```python
from build123d import *
from OCP.BRepFilletAPI import BRepFilletAPI_MakeChamfer

# Parameters (mm, degrees)
SKETCH1_R           = 1.5
BOSS_EXTRUDE1_DEPTH = 50
SKETCH2_W           = 6
SKETCH2_H           = 50
BOSS_EXTRUDE2_DEPTH = 50
CHAMFER1_SIZE       = 50
CHAMFER1_SIZE2      = 20
SKETCH4_W           = 6
SKETCH4_H           = 3
BOSS_EXTRUDE3_DEPTH = 6
SKETCH5_R           = 1.5
CUT_EXTRUDE1_DEPTH  = 65.747586828
CHAMFER2_SIZE       = 1
CHAMFER2_SIZE2      = 1.795054936
FILLET1_R           = 2
CUT_EXTRUDE2_DEPTH  = 6
CUT_EXTRUDE3_DEPTH  = 78.569323834
BOSS_EXTRUDE5_DEPTH = 6
CUT_EXTRUDE4_DEPTH  = 78.569323834
FILLET2_R           = 10


with BuildPart() as part:
    # Sketch1 → Boss-Extrude1 (new body)
    with BuildSketch(Plane(origin=(0, 0, 0), x_dir=(1, 0, 0), z_dir=(0, 1, 0))):
        with BuildLine():
            Line((0, 3), (-3, 3))
            Line((-3, 3), (-3, -3))
            Line((-3, -3), (0, -3))
            ThreePointArc((0, -3), (3, 0), (0, 3))
        make_face()
        with Locations(Location((0, 0, 0), (0, 0, 270))):
            Circle(SKETCH1_R, mode=Mode.SUBTRACT)
    extrude(amount=BOSS_EXTRUDE1_DEPTH)

    # Sketch2 → Boss-Extrude2 (add)
    with BuildSketch(Plane.ZY.offset(3)):
        with Locations((0, 25)):
            Rectangle(SKETCH2_W, SKETCH2_H)
    extrude(amount=BOSS_EXTRUDE2_DEPTH)

    # Chamfer1: one chamfer whose edges measure the first distance from different faces: ONE call of the kernel's chamfer builder (chamfer() names one face for all edges)
    chamfer1_edges_1 = [part.edges().sort_by_distance(p)[0] for p in [
        (-53, 50, 0),
    ]]
    chamfer1_side_1 = [part.faces().sort_by_distance(p)[0] for p in [
        (-25.86838725, 50, 0),
    ]]
    chamfer1_edges_2 = [part.edges().sort_by_distance(p)[0] for p in [
        (-53, 0, 0),
    ]]
    chamfer1_side_2 = [part.faces().sort_by_distance(p)[0] for p in [
        (-25.86838725, 0, 0),
    ]]
    chamfer1 = BRepFilletAPI_MakeChamfer(part.part.solid().wrapped)
    for e in chamfer1_edges_1:
        chamfer1.Add(CHAMFER1_SIZE, CHAMFER1_SIZE2, e.wrapped, chamfer1_side_1[0].wrapped)  # the first distance lies on this face
    for e in chamfer1_edges_2:
        chamfer1.Add(CHAMFER1_SIZE, CHAMFER1_SIZE2, e.wrapped, chamfer1_side_2[0].wrapped)  # the first distance lies on this face
    add(Compound.cast(chamfer1.Shape()), mode=Mode.REPLACE)

    # Sketch4 → Boss-Extrude3 (add)
    with BuildSketch(Plane.ZY.offset(53)):
        with Locations((0, 25)):
            Rectangle(SKETCH4_W, SKETCH4_H)
    extrude(amount=BOSS_EXTRUDE3_DEPTH)

    # Sketch5 → Cut-Extrude1 (cut, through all)
    with BuildSketch(Plane.XZ.offset(-23.5)):
        with Locations(Location((-56, 0, 0), (0, 0, 270))):
            Circle(SKETCH5_R)
    extrude(amount=-CUT_EXTRUDE1_DEPTH, mode=Mode.SUBTRACT)

    # Chamfer2: one chamfer whose edges measure the first distance from different faces: ONE call of the kernel's chamfer builder (chamfer() names one face for all edges)
    chamfer2_edges_1 = [part.edges().sort_by_distance(p)[0] for p in [
        (-53, 30, 0),
    ]]
    chamfer2_side_1 = [part.faces().sort_by_distance(p)[0] for p in [
        (-28, 40, 0),
    ]]
    chamfer2_edges_2 = [part.edges().sort_by_distance(p)[0] for p in [
        (-53, 20, 0),
    ]]
    chamfer2_side_2 = [part.faces().sort_by_distance(p)[0] for p in [
        (-28, 10, 0),
    ]]
    chamfer2 = BRepFilletAPI_MakeChamfer(part.part.solid().wrapped)
    for e in chamfer2_edges_1:
        chamfer2.Add(CHAMFER2_SIZE, CHAMFER2_SIZE2, e.wrapped, chamfer2_side_1[0].wrapped)  # the first distance lies on this face
    for e in chamfer2_edges_2:
        chamfer2.Add(CHAMFER2_SIZE, CHAMFER2_SIZE2, e.wrapped, chamfer2_side_2[0].wrapped)  # the first distance lies on this face
    add(Compound.cast(chamfer2.Shape()), mode=Mode.REPLACE)

    # Fillet1
    fillet1_edges = [part.edges().sort_by_distance(p)[0] for p in [
        (-59, 25, 3),
        (-59, 25, -3),
    ]]
    fillet(fillet1_edges, radius=FILLET1_R)

    # Sketch6 → Cut-Extrude2 (cut)
    with BuildSketch(Plane.XY.offset(3)):
        Polygon((-7.907152331, 5), (-5.507152331, 5), (-5.507152331, 45), (-7.907152331, 45), (-47.164370978, 29.297112541), (-47.907152331, 27.563956051), (-47.907152331, 22.436043949), (-47.164370978, 20.702887459), align=None)
    extrude(amount=-CUT_EXTRUDE2_DEPTH, mode=Mode.SUBTRACT)

    # Sketch7 → Cut-Extrude3 (cut, through all)
    with BuildSketch(Plane.XY.offset(3)):
        Polygon((-53, 28.204945064), (-53, 26.5), (-47.907152331, 26.5), (-47.907152331, 27.563956051), (-47.164370978, 29.297112541), (-25.810496084, 37.838662499), (-14.112413915, 45.555034434), (-52.071523309, 30.371390676), align=None)
        Polygon((-47.907152331, 23.5), (-53, 23.5), (-53, 21.795054936), (-52.071523309, 19.628609324), (-14.112413915, 4.444965566), (-25.810496084, 12.161337501), (-47.164370978, 20.702887459), (-47.907152331, 22.436043949), align=None)
    extrude(amount=-CUT_EXTRUDE3_DEPTH, mode=Mode.SUBTRACT)


with BuildPart() as cut_extrude3_piece_1:
    # of the separate pieces the step leaves, piece 1, a body of its own (cut_extrude3_pieces)
    add(part.part.solids().sort_by_distance((-3, 50, -3))[0])



with BuildPart() as cut_extrude3_piece_2:
    # of the separate pieces the step leaves, piece 2, a body of its own (cut_extrude3_pieces)
    add(part.part.solids().sort_by_distance((-57, 26.5, -3))[0])


with BuildPart() as cut_extrude3_piece_1_1:
    add(cut_extrude3_piece_1.part)

    add(cut_extrude3_piece_2.part)  # Boss-Extrude5 merges Cut-Extrude3 piece 2
    # Sketch7<3> → Boss-Extrude5 (add)
    with BuildSketch(Plane.XY.offset(3)):
        Polygon((-43, 26.5), (-53, 26.5), (-53, 23.5), (-43, 23.5), (-14.112413915, 4.444965566), (-3, 0), (-3, 50), (-14.112413915, 45.555034434), align=None)
    extrude(amount=-BOSS_EXTRUDE5_DEPTH)

    # Sketch8 → Cut-Extrude4 (cut, through all)
    with BuildSketch(Plane.XY.offset(3)):
        Polygon((-35.341555741, 26.05), (-15.120245482, 39.388524104), (-7.341555741, 42.5), (-5.241555741, 42.5), (-5.241555741, 7.5), (-7.341555741, 7.5), (-15.120245482, 10.611475896), (-35.341555741, 23.95), align=None)
    extrude(amount=-CUT_EXTRUDE4_DEPTH, mode=Mode.SUBTRACT)

    # Fillet2
    fillet2_edges = [cut_extrude3_piece_1_1.edges().sort_by_distance(p)[0] for p in [
        (-43, 23.5, 0),
        (-43, 26.5, 0),
    ]]
    fillet(fillet2_edges, radius=FILLET2_R)


solid = cut_extrude3_piece_1_1.part
```
Design review of the part built by this model. Coordinates are the model's own, in mm. A direction names the side the tool comes from. Give positions to 0.01 mm unless a question says otherwise; leave off trailing zeros. Write each loop counter-clockwise with the first axis right and the second up, starting at its lowest first coordinate (ties: lowest second). Pieces come first, ordered by that corner, then holes. Notation, with made-up numbers: (39, -29.75) -> (60, -29.75) arc R23 ccw to (60, -11.75) -> close; hole circle Ø8 at (-24, -27.5). An arc over 180 degrees is marked (long way). Answer in a Markdown table with one row per item.
(1) Consider section D-D (y = 44.5). State the section outline as (x, z) points, then the cut area to 3 significant figures.
Results:
| item | result |
|---|---|
| outline | (-15.71, -3) -> (0, -3) arc R3 ccw to (0, 3) -> (-15.71, 3) -> close; hole circle Ø3 at (0, 0) |
| area | 101 mm2 |
(2) Mouldability with a two-part tool opening along Y and no side actions: class faces 5 (the flat face through (-25.372, 32.626, 0.042)), 6 (the flat face through (-8.63, 47.75, -0.04)), 7 (the flat face through (-59, 25, 0)) as +Y half, -Y half, draft (parallel to the pull), parting line (faces both ways), or undercut.
Results:
| item | result |
|---|---|
| face 5 | undercut |
| face 6 | +Y half |
| face 7 | draft |
(3) For faces 1 (the flat face through (-52, 26.5, 0)), 2 (the flat face through (-11.29, 40.92, 0.04)), 3 (the flat face through (-53, 23.5, 0)), 4 (the cylindrical face through (-58.4, 25.02, -2.43)), list the 3-axis set-ups (+Z, -Z, +X, -X, +Y, -Y) from which the entire face can be reached by the end or side of a thin tool; tool diameter is ignored.
Results:
| item | result |
|---|---|
| face 1 | +Z, -Z, -X, +Y |
| face 2 | +Z, -Z |
| face 3 | +Z, -Z, -X, -Y |
| face 4 | -Z, -X, +Y, -Y |
(4) Consider section A-A (z = 0). State the section outline as (x, y) points, then the cut area to 3 significant figures.
Results:
| item | result |
|---|---|
| outline | (-59, 23.5) -> (-57.5, 23.5) -> (-57.5, 26.5) -> (-59, 26.5) -> close; (-54.5, 23.5) -> (-46, 23.5) arc R10 cw to (-40.49, 21.85) -> (-14.11, 4.44) -> (-3, 0) -> (-1.5, 0) -> (-1.5, 50) -> (-3, 50) -> (-14.11, 45.56) -> (-40.49, 28.15) arc R10 cw to (-46, 26.5) -> (-54.5, 26.5) -> close; (1.5, 0) -> (3, 0) -> (3, 50) -> (1.5, 50) -> close; hole (-35.34, 23.95) -> (-15.12, 10.61) -> (-7.34, 7.5) -> (-5.24, 7.5) -> (-5.24, 42.5) -> (-7.34, 42.5) -> (-15.12, 39.39) -> (-35.34, 26.05) -> close |
| area | 700 mm2 |
(5) Consider section B-B (x = -56). State the section outline as (y, z) points, then the cut area to 3 significant figures.
Results:
| item | result |
|---|---|
| outline | (23.5, -3) -> (26.5, -3) -> (26.5, -1.5) -> (23.5, -1.5) -> close; (23.5, 1.5) -> (26.5, 1.5) -> (26.5, 3) -> (23.5, 3) -> close |
| area | 9.00 mm2 |
(6) To check wall thickness, follow probe 1 along X at (y, z) = (28, 0); probe 2 along X at (y, z) = (18, 0.5); probe 3 along Y at (x, z) = (-48, -2.25). State the ranges of each line that lie inside material, in increasing order.
Results:
| item | result |
|---|---|
| probe 1 | -40.73 to -32.39, -5.24 to -1.5, 1.5 to 3 |
| probe 2 | -34.66 to -26.32, -5.24 to -1.41, 1.41 to 2.96 |
| probe 3 | 23.5 to 26.5 |
(7) Consider section C-C (y = 14). State the section outline as (x, z) points.
Results:
| item | result |
|---|---|
| outline | (-28.6, -3) -> (-20.26, -3) -> (-20.26, 3) -> (-28.6, 3) -> close; (-5.24, -3) -> (0, -3) arc R3 ccw to (0, 3) -> (-5.24, 3) -> close; hole circle Ø3 at (0, 0) |
(8) Clearance check with flat-ended pins moving along their axes: pin 1 (0.6 mm diameter, centred on x = -6.5, z = -0.5, fed in from +Y); pin 2 (1.7 mm diameter, centred on x = -6.5, z = 1, fed in from -Y); pin 3 (1.5 mm diameter, centred on x = -28, z = 2, fed in from -Y). State where each tip first meets the part, or that it passes through.
Results:
| item | result |
|---|---|
| pin 1 | y = 48.72 |
| pin 2 | y = 1.06 |
| pin 3 | y = 13.11 |
